Check sheet for the drawn part. Datum: minimum x, y, z corner. Units: mm. Give positions to 0.01 mm unless a question says otherwise; leave off trailing zeros. Write each loop counter-clockwise with the first axis right and the second up, starting at its lowest first coordinate (ties: lowest second). Pieces come first, ordered by that corner, then holes. Notation, with made-up numbers: M 23.25,58 L 36.25,58 A31 ccw 36.25,91 Z; hole C 3,76.5 d3. An arc over 180 degrees is marked long. Write item = value, one per line.
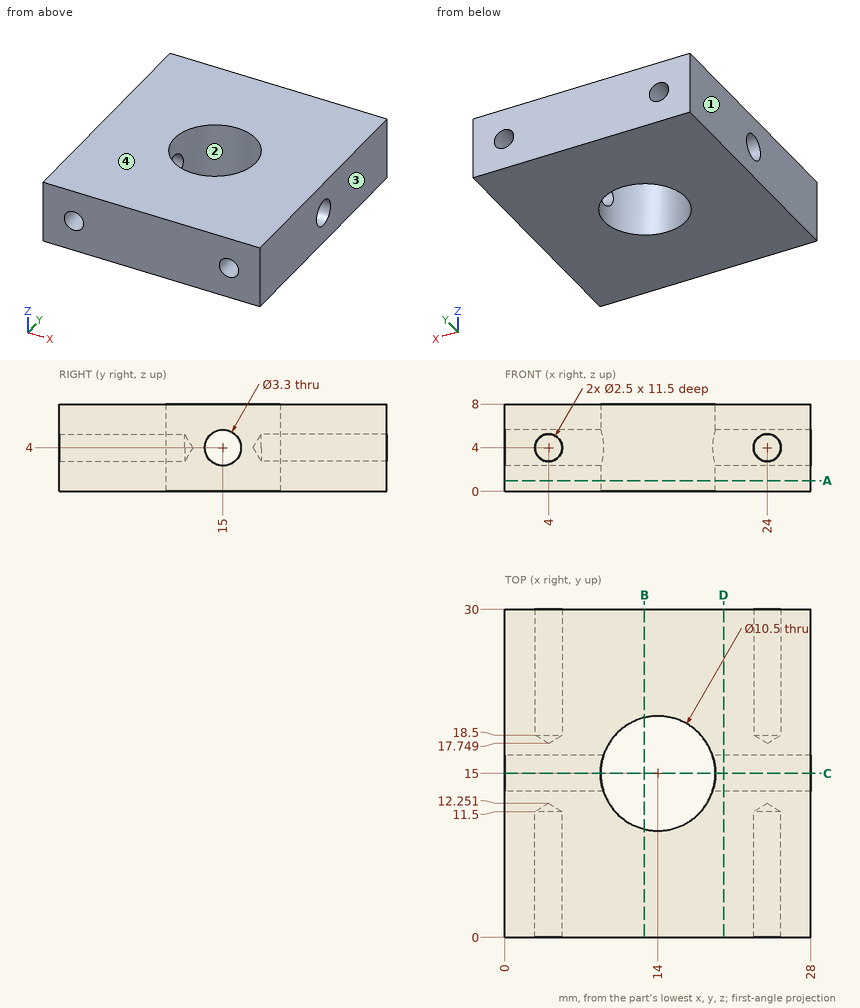
1) Cross-section at B-B on x = 12.75. Record the boundary of the cut face in (y, z).
From the geometry:
outline = M 0,0 L 9.9,0 L 9.9,8 L 0,8 Z; M 20.1,0 L 30,0 L 30,8 L 20.1,8 Z
2) Depth check by flat-ended pin: P1, Ø2, axis at x = 24, z = 4, coming from the +Y side; P2, Ø1.5, axis at x = 6, z = 4.5, coming from the -Y side; P3, Ø8.5, axis at x = 14, y = 15, coming from the -Z side; P4, Ø2, axis at x = 24, z = 4, coming from the -Y side. Enter the tip coordinate at first touch or a pass-through.
From the geometry:
P1 = 18.35
P2 = 0
P3 = through
P4 = 11.65
3) Material ranges on probe 1 along Z at (x, y) = (3.25, 15); probe 2 along Z at (x, y) = (24, 22); probe 3 along X at (y, z) = (1.75, 5), recorded low to high. Write a range as from..to.
From the geometry:
probe_1 = 0..2.35, 5.65..8
probe_2 = 0..2.75, 5.25..8
probe_3 = 0..3.25, 4.75..23.25, 24.75..28
4) Draft check along X on the marked faces 1, 2, 3 and 4. Enter one of: +X half, -X half, draft (parallel to the pull), parting line (faces both ways), or undercut.
From the geometry:
face_1 = -X half
face_2 = undercut
face_3 = +X half
face_4 = draft
5) Cross-section at A-A on z = 1. Record the boundary of the cut face in (x, y).
From the geometry:
outline = M 0,0 L 28,0 L 28,30 L 0,30 Z; hole C 14,15 d10.5
6) Cross-section at C-C on y = 15. Record the boundary of the cut face in (x, z).
From the geometry:
outline = M 0,0 L 8.75,0 L 8.75,2.35 L 0,2.35 Z; M 0,5.65 L 8.75,5.65 L 8.75,8 L 0,8 Z; M 19.25,0 L 28,0 L 28,2.35 L 19.25,2.35 Z; M 19.25,5.65 L 28,5.65 L 28,8 L 19.25,8 Z
7) Cross-section at D-D on x = 20. Record the boundary of the cut face in (y, z).
From the geometry:
outline = M 0,0 L 30,0 L 30,8 L 0,8 Z; hole C 15,4 d3.3
